Can you work these out from the model? Positions are in its coordinate system, mm. Face numbers are marked on the shaded views. Round coordinates to 2 decimals unless told otherwise and drop trailing zeros. Order: outer loops, then holes, each group sorted by start corner. A loop starts at its lowest first (then second) coordinate and runs counter-clockwise, first axis right, second up.
from build123d import *

# Parameters (mm, degrees)
ESQUISSE1_W             = 4
ESQUISSE1_H             = 20
BOSS_EXTRU_1_DEPTH      = 3
ESQUISSE3_R             = 1
ENL_V_MAT_EXTRU_1_DEPTH = 6
CONG_4_R                = 1
CONG_5_R                = 1
CONG_6_R                = 1
CONG_7_R                = 1


with BuildPart() as part:
    # Esquisse1 → Boss.-Extru.1 (new body)
    with BuildSketch(Plane.XY):
        with Locations((2, 10)):
            Rectangle(ESQUISSE1_W, ESQUISSE1_H)
    extrude(amount=BOSS_EXTRU_1_DEPTH)

    # Esquisse3 → Enlèv. mat.-Extru.1 (cut)
    with BuildSketch(Plane.XY.offset(3)):
        with Locations((2, 2)):
            Circle(ESQUISSE3_R)
        with Locations((2, 18)):
            Circle(ESQUISSE3_R)
    extrude(amount=-ENL_V_MAT_EXTRU_1_DEPTH, mode=Mode.SUBTRACT)

    # Congé4
    cong_4_edges = [part.edges().sort_by_distance(p)[0] for p in [
        (4, 0, 1.5),
    ]]
    fillet(cong_4_edges, radius=CONG_4_R)

    # Congé5
    cong_5_edges = [part.edges().sort_by_distance(p)[0] for p in [
        (0, 0, 1.5),
    ]]
    fillet(cong_5_edges, radius=CONG_5_R)

    # Congé6
    cong_6_edges = [part.edges().sort_by_distance(p)[0] for p in [
        (0, 20, 1.5),
    ]]
    fillet(cong_6_edges, radius=CONG_6_R)

    # Congé7
    cong_7_edges = [part.edges().sort_by_distance(p)[0] for p in [
        (4, 20, 1.5),
    ]]
    fillet(cong_7_edges, radius=CONG_7_R)


solid = part.part
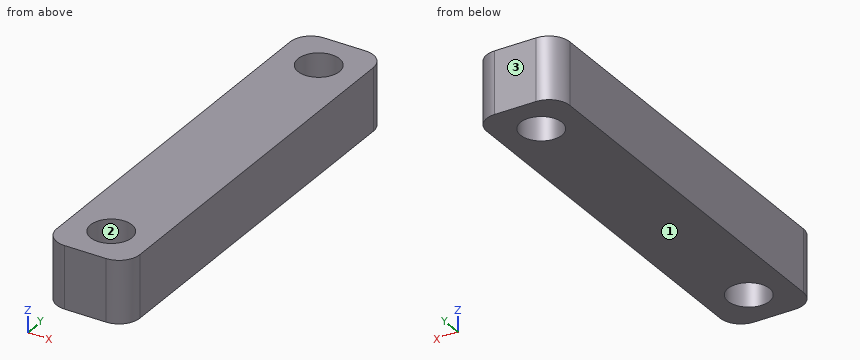
(1) If we mould it in two halves opening along Y, with no side actions, what happens to the marked faces 1, 2 and 3? For each: pulls with the +Y half, pulls with the -Y half, needs draft (parallel to the pull), parting line crosses it, or undercut.
(2) Please list where these lines run through material, in increasing order: probe 1 along Y at (x, z) = (2, 1.85); probe 2 along Y at (x, z) = (2.7, 1.05); probe 3 along X at (y, z) = (1.25, 1.9).
(3) I want a section at C-C, the plane z = 0.2. List the corners of the cut face in (x, y) for me.
(4) I want a section at B-B, the plane y = 18. List the corners of the cut face in (x, z) for me.
(5) I want a section at A-A, the plane x = 2.6. List the corners of the cut face in (y, z) for me, plus the area to 3 significant figures.
(6) I want a section at D-D, the plane x = 1.2. List the corners of the cut face in (y, z) for me, plus the area to 3 significant figures.
Ans:
1. face 1: needs draft
1. face 2: undercut
1. face 3: pulls with the +Y half
2. probe 1: y = 0 to 1, 3 to 17, 19 to 20
2. probe 2: y = 0 to 1.29, 2.71 to 17.29, 18.71 to 20
2. probe 3: x = 0 to 1.34, 2.66 to 4
3. outline: (0, 1) arc R1 ccw to (1, 0) - (3, 0) arc R1 ccw to (4, 1) - (4, 19) arc R1 ccw to (3, 20) - (1, 20) arc R1 ccw to (0, 19) - close; hole circle Ø2 at (2, 2); hole circle Ø2 at (2, 18)
4. outline: (0, 0) - (1, 0) - (1, 3) - (0, 3) - close; (3, 0) - (4, 0) - (4, 3) - (3, 3) - close
5. outline: (0, 0) - (1.2, 0) - (1.2, 3) - (0, 3) - close; (2.8, 0) - (17.2, 0) - (17.2, 3) - (2.8, 3) - close; (18.8, 0) - (20, 0) - (20, 3) - (18.8, 3) - close
5. area: 50.4 mm2
6. outline: (0, 0) - (1.4, 0) - (1.4, 3) - (0, 3) - close; (2.6, 0) - (17.4, 0) - (17.4, 3) - (2.6, 3) - close; (18.6, 0) - (20, 0) - (20, 3) - (18.6, 3) - close
6. area: 52.8 mm2
